```python
from build123d import *

# Parameters (mm, degrees)
F0_W     = 50.8
F0_H     = 50.8
F1_DEPTH = 50.8
F2_W     = 45.72
F2_H     = 45.72
F3_DEPTH = 50.8
F4_W     = 45.72
F4_H     = 45.72
F5_DEPTH = 50.8
F6_W     = 45.72
F6_H     = 45.72
F7_DEPTH = 50.8


with BuildPart() as f1:
    # F0 (on Top) → F1 (new body)
    with BuildSketch(Plane.XY):
        with Locations((25.4, -25.4)):
            Rectangle(F0_W, F0_H)
    extrude(amount=F1_DEPTH)

    # F2 (on face) → F3 (cut)
    with BuildSketch(Plane.XY.offset(50.8)):
        with Locations((25.4, -25.4)):
            Rectangle(F2_W, F2_H)
    extrude(amount=-F3_DEPTH, mode=Mode.SUBTRACT)

    # F4 (on face) → F5 (cut)
    with BuildSketch(Plane.XZ.offset(50.8)):
        with Locations((25.4, 25.4)):
            Rectangle(F4_W, F4_H)
    extrude(amount=-F5_DEPTH, mode=Mode.SUBTRACT)

    # F6 (on face) → F7 (cut)
    with BuildSketch(Plane.YZ.offset(50.8)):
        with Locations((-25.4, 25.4)):
            Rectangle(F6_W, F6_H)
    extrude(amount=-F7_DEPTH, mode=Mode.SUBTRACT)


solid = f1.part
```
Design review of the part built by this model. Coordinates are the model's own, in mm. A direction names the side the tool comes from. Give positions to 0.01 mm unless a question says otherwise; leave off trailing zeros. Order: outer loops, then holes, each group sorted by start corner. A loop starts at its lowest first (then second) coordinate and runs counter-clockwise, first axis right, second up. Notation, with made-up numbers: M 1,-0.75 L 43,-0.75 A24 ccw 43,27.25 Z; hole C 60.5,7.5 d10. An arc over 180 degrees is marked long. One line per question, with ' | ' between items. Start each with the question number.
Q1. We need section A-A (x = 33). Write out the cut boundary in (y, z), plus the area to 3 significant figures.
Q2. We need section B-B (z = 9.5). Write out the cut boundary in (x, y), plus the area to 3 significant figures.
Q3. For pin 1 Ø1.3 at (x, y) = (50, -35) entering from -Z, flat-tipped, find the tip position at first contact; note if it passes through.
Q4. Machinability: for faces 1 (the face through (23, -50.8, 50)), 2 (the face through (48.26, -50, 25)), 3 (the face through (48.26, -26, 1)), 4 (the face through (0, -27, 50)), 5 (the face through (50, -2.54, 25)), which of the approach directions +Z, -Z, +X, -X, +Y, -Y give a long, thin tool a straight path to every point of the face, cutting with its end or side? Answer none if there is none.
Q5. The part is to be moulded in two halves that separate along Z. For faces 6 (the face through (2.54, -50, 25)), 7 (the face through (2.54, -26, 1)), 8 (the face through (23, -50, 50.8)), say which applies: +Z half, -Z half, draft (parallel to the pull), parting line (faces both ways), or undercut.
Returned:
1) outline: M -50.8,0 L -48.26,0 L -48.26,2.54 L -50.8,2.54 Z; M -50.8,48.26 L -48.26,48.26 L -48.26,50.8 L -50.8,50.8 Z; M -2.54,0 L 0,0 L 0,2.54 L -2.54,2.54 Z; M -2.54,48.26 L 0,48.26 L 0,50.8 L -2.54,50.8 Z | area: 25.8 mm2
2) outline: M 0,-50.8 L 2.54,-50.8 L 2.54,-48.26 L 0,-48.26 Z; M 0,-2.54 L 2.54,-2.54 L 2.54,0 L 0,0 Z; M 48.26,-50.8 L 50.8,-50.8 L 50.8,-48.26 L 48.26,-48.26 Z; M 48.26,-2.54 L 50.8,-2.54 L 50.8,0 L 48.26,0 Z | area: 25.8 mm2
3) pin 1: z = 0
4) face 1: +Z, -Z, +X, -X, -Y | face 2: +Y, -Y | face 3: +Z, -Z | face 4: +Z, -Z, -X, +Y, -Y | face 5: +X, -X
5) face 6: undercut | face 7: draft | face 8: +Z half
